```python
from build123d import *

# Parameters (mm, degrees)
SKETCH1_W           = 50.8
SKETCH1_H           = 25.4
SKETCH1_W_2         = 47.9
SKETCH1_H_2         = 22.5
BOSS_EXTRUDE1_DEPTH = 457.2
SKETCH2_R           = 2.5
CUT_EXTRUDE1_DEPTH  = 459.608940166


with BuildPart() as part:
    # Sketch1 → Boss-Extrude1 (new body)
    with BuildSketch(Plane(origin=(0, 0, 0), x_dir=(1, 0, 0), z_dir=(0, 1, 0))):
        Rectangle(SKETCH1_W, SKETCH1_H)
        Rectangle(SKETCH1_W_2, SKETCH1_H_2, mode=Mode.SUBTRACT)
    extrude(amount=BOSS_EXTRUDE1_DEPTH)

    # Sketch2 → Cut-Extrude1 (cut, through all)
    with BuildSketch(Plane.XY.offset(12.7)):
        with Locations((-11.25, 60)):
            Circle(SKETCH2_R)
        with Locations((-11.25, 25)):
            Circle(SKETCH2_R)
        with Locations((11.25, 25)):
            Circle(SKETCH2_R)
        with Locations((11.25, 60)):
            Circle(SKETCH2_R)
    cut_extrude1 = extrude(amount=-CUT_EXTRUDE1_DEPTH, mode=Mode.SUBTRACT)

    # Mirror1: Cut-Extrude1 across plane
    add(cut_extrude1.mirror(Plane.ZX.offset(228.6)), mode=Mode.SUBTRACT)


solid = part.part
```
Read the model definition and answer for the solid it produces. Units are mm, in the model's axes. A direction names the side the tool comes from. Give positions to 0.01 mm unless a question says otherwise; leave off trailing zeros. Loops run counter-clockwise (first coordinate to the right, second up) from the corner with the lowest first, then second, coordinate; pieces in that order, holes last.
Item 1: The part is cut by section A-A (z = -7). Write down the section's boundary in (x, y), and give its area (3 significant figures).
Item 2: The part is cut by section B-B (x = -5). Write down the section's boundary in (y, z), and give its area (3 significant figures).
Item 3: The mould has two halves that part along Z. Classify faces 1 (the flat face through (23.95, 225, 0)), 2 (the flat face through (0, 225, 12.7)), 3 (the flat face through (-25.4, 225, 0)), 4 (the flat face through (0, 225, -12.7)): released by +Z, released by -Z, zero draft, split by the parting line, or undercut.
Item 4: Find the intervals of material crossed by line 1 along X through (y, z) = (432.2, 12.05); line 2 along Z through (x, y) = (4, 358); line 3 along X through (y, z) = (202, -6.5), in increasing order.
Item 5: Each of these flat-tipped pins is pushed along its axis until it touches: pin 1 Ø6 at (x, y) = (-11.25, 60) entering from -Z; pin 2 Ø3 at (x, y) = (11.25, 432.2) entering from -Z. Where does it stop, or does it pass through?
Item 6: The part is cut by section C-C (y = 321). Write down the section's boundary in (x, z).
Item 7: For faces 5 (the flat face through (0, 225, -11.25)), 6 (the flat face through (25.4, 225, 0)), determine the directions among +Z, -Z, +X, -X, +Y, -Y from which every point of the face is accessible in a straight line to the end or side of a thin tool.
Taken from the geometry:
1. outline: (-25.4, 0) - (-23.95, 0) - (-23.95, 457.2) - (-25.4, 457.2) - close; (23.95, 0) - (25.4, 0) - (25.4, 457.2) - (23.95, 457.2) - close
1. area: 1,330 mm2
2. outline: (0, -12.7) - (457.2, -12.7) - (457.2, -11.25) - (0, -11.25) - close; (0, 11.25) - (457.2, 11.25) - (457.2, 12.7) - (0, 12.7) - close
2. area: 1,330 mm2
3. face 1: undercut
3. face 2: released by +Z
3. face 3: zero draft
3. face 4: released by -Z
4. line 1: x = -25.4 to -13.75, -8.75 to 8.75, 13.75 to 25.4
4. line 2: z = -12.7 to -11.25, 11.25 to 12.7
4. line 3: x = -25.4 to -23.95, 23.95 to 25.4
5. pin 1: stops at z = -12.7
5. pin 2: passes through
6. outline: (-25.4, -12.7) - (25.4, -12.7) - (25.4, 12.7) - (-25.4, 12.7) - close; hole (-23.95, -11.25) - (23.95, -11.25) - (23.95, 11.25) - (-23.95, 11.25) - close
7. face 5: +Y, -Y
7. face 6: +Z, -Z, +X, +Y, -Y
